Geometry check sheet. Reference: the model listing, model coordinates, mm. A direction names the side the tool comes from. Round coordinates to 2 decimals unless told otherwise and drop trailing zeros. Write each loop counter-clockwise with the first axis right and the second up, starting at its lowest first coordinate (ties: lowest second). Pieces come first, ordered by that corner, then holes. Notation, with made-up numbers: (20.25, 45) - (52.25, 45) arc R33 cw to (52.25, 77) - close; hole circle Ø10 at (85.25, -36). An arc over 180 degrees is marked (long way). Return JSON: item names as keys, results as strings.
Autodesk Inventor part; units mm, degrees
ref_plane "YZ Plane" through (0, 0, 0) normal (1, 0, 0) x (0, 1, 0)
ref_plane "XZ Plane" through (0, 0, 0) normal (0, 1, 0) x (-1, 0, 0)
ref_plane "XY Plane" through (0, 0, 0) normal (0, 0, 1) x (1, 0, 0)
sketch "Sketch1" plane through (0, 0, 0) normal (0, 0, 1) x (1, 0, 0)
  line L0 (0, 35.9415) -> (0, -22.75) construction
  line L1 (5, 30) -> (15, 30)
  line L2 (15, 30) -> (15, -30)
  line L3 (15, -30) -> (5, -30)
  line L4 (5, -30) -> (5, 30)
  circle A0 centre (10, 25) radius 2.25
  circle A1 centre (10, -25) radius 2.25
  line L5 (-5, 22.5) -> (5, 22.5)
  line L6 (5, 22.5) -> (5, -22.5)
  line L7 (5, -22.5) -> (-5, -22.5)
  line L8 (-5, -22.5) -> (-5, 22.5)
  line L9 (-5, 22.5) -> (5, 22.5)
  line L10 (5, 22.5) -> (5, 16.5)
  line L11 (5, 16.5) -> (-5, 16.5)
  line L12 (-5, 16.5) -> (-5, 22.5)
  line L13 (-5, -22.5) -> (5, -22.5)
  line L14 (5, -22.5) -> (5, -16.5)
  line L15 (5, -16.5) -> (-5, -16.5)
  line L16 (-5, -16.5) -> (-5, -22.5)
  line L17 (-5, 3) -> (5, 3)
  line L18 (5, 3) -> (5, -3)
  line L19 (5, -3) -> (-5, -3)
  line L20 (-5, -3) -> (-5, 3)
  point P0 (0, 0)
  point P1 (15, 0)
  point P2 (5, 0)
  point P3 (0, 22.5)
  point P4 (5, 0)
  point P5 (5, 0)
  dimension "d28" = 60
  dimension "d29" = 4.5
  dimension "d30" = 4.5
  dimension "d31" = 5
  dimension "d32" = 5
  dimension "d33" = 10
  dimension "d36" = 10
  dimension "d37" = 45
  dimension "d38" = 5
  dimension "d39" = 5
  dimension "d42" = 6
  dimension "d43" = 6
  dimension "d44" = 6
extrude "Extrusion3" add sketch "Sketch1" along normal blind 1.8 contours L4 L11 L8 L5 | L4 L17 L8 L11 | L4 L19 L8 L17 | L7 L8 L15 L4 | L4 L15 L8 L19
extrude "Extrusion5" add sketch "Sketch1" along normal blind 2.4 contours L1 L2 L3 L4
extrude "Extrusion6" add sketch "Sketch1" along normal blind 2.4 contours L4 L11 L8 L5 | L4 L19 L8 L17 | L7 L8 L15 L4
mirror "Mirror2" about plane through (0, 0, 0) normal (1, 0, 0) of "Extrusion5", "Extrusion6"
equation "\"d29\" = screw"
equation "\"d30\" = screw"
properties part number "FoldLink" material "Rubber, Silicone"
(1) Material ranges on line 1 along Y through (x, z) = (10, 1.1); line 2 along Y through (x, z) = (11, 1.35); line 3 along X through (y, z) = (26, 2.1), recorded low to high. Write a range as [from, to].
Response values:
{"line 1": "y = [-30, -27.25], [-22.75, 22.75], [27.25, 30]", "line 2": "y = [-30, -27.02], [-22.98, 22.98], [27.02, 30]", "line 3": "x = [-15, -12.02], [-7.98, -5], [5, 7.98], [12.02, 15]"}
(2) Section check C-C, the plane z = 1.05. Enter the section's corners in (x, y).
Response values:
{"outline": "(-15, -30) - (-5, -30) - (-5, -22.5) - (5, -22.5) - (5, -30) - (15, -30) - (15, 30) - (5, 30) - (5, 22.5) - (-5, 22.5) - (-5, 30) - (-15, 30) - close; hole circle Ø4.5 at (-10, -25); hole circle Ø4.5 at (-10, 25); hole circle Ø4.5 at (10, -25); hole circle Ø4.5 at (10, 25)"}
(3) Section check A-A, the plane x = -10. Enter the section's corners in (y, z).
Response values:
{"outline": "(-30, 0) - (-27.25, 0) - (-27.25, 2.4) - (-30, 2.4) - close; (-22.75, 0) - (22.75, 0) - (22.75, 2.4) - (-22.75, 2.4) - close; (27.25, 0) - (30, 0) - (30, 2.4) - (27.25, 2.4) - close"}
(4) Access from +Z, -Z, +X, -X, +Y, -Y to the whole of each face (thin tool, end or side, straight path). Record for faces 1 (the face through (0, -22.5, 1)), 2 (the face through (5, 26, 1)), 3 (the face through (0, -10, 1.8)).
Response values:
{"face 1": "+Z, -Z, -Y", "face 2": "+Z, -Z, +Y", "face 3": "+Z"}
(5) Section check D-D, the plane y = 24. Enter the section's corners in (x, z), plus the area to 3 significant figures.
Response values:
{"outline": "(-15, 0) - (-12.02, 0) - (-12.02, 2.4) - (-15, 2.4) - close; (-7.98, 0) - (-5, 0) - (-5, 2.4) - (-7.98, 2.4) - close; (5, 0) - (7.98, 0) - (7.98, 2.4) - (5, 2.4) - close; (12.02, 0) - (15, 0) - (15, 2.4) - (12.02, 2.4) - close", "area": "28.7 mm^2"}
(6) Section check B-B, the plane y = -25. Enter the section's corners in (x, z), plus the area to 3 significant figures.
Response values:
{"outline": "(-15, 0) - (-12.25, 0) - (-12.25, 2.4) - (-15, 2.4) - close; (-7.75, 0) - (-5, 0) - (-5, 2.4) - (-7.75, 2.4) - close; (5, 0) - (7.75, 0) - (7.75, 2.4) - (5, 2.4) - close; (12.25, 0) - (15, 0) - (15, 2.4) - (12.25, 2.4) - close", "area": "26.4 mm^2"}
(7) Gauge pin test, flat end, axial feed: pin 1 (0.5 mm diameter, centred on x = -0.5, z = 2, fed in from -Y). Record the tip position at first contact, or that the pin passes through.
Response values:
{"pin 1": "stops at y = -22.5"}
(8) Release check for a two-part mould opening along Y. For faces 4 (the face through (-10, 30, 1)), 5 (the face through (0, 10, 1.8)), 6 (the face through (-5, 26, 1)) record: pulls with the +Y half, pulls with the -Y half, needs draft (parallel to the pull), parting line crosses it, or undercut.
Response values:
{"face 4": "pulls with the +Y half", "face 5": "undercut", "face 6": "needs draft"}
